from build123d import *

# Parameters (mm, degrees)
SKETCH_1_W          = 32.4
SKETCH_1_H          = 30
EXTRUDE_1_DEPTH     = 1.5
SKETCH_2_W          = 4.9
SKETCH_2_H          = 8.52
EXTRUDE_2_DEPTH     = 10
CUT_EXTRUDE_1_DEPTH = 11.5
SKETCH_4_R          = 1
CUT_EXTRUDE_2_DEPTH = 31.5
CUT_EXTRUDE_3_DEPTH = 10
EXTRUDE_3_DEPTH     = 2
CUT_EXTRUDE_4_DEPTH = 6
SKETCH_8_R          = 2.25
CUT_EXTRUDE_5_DEPTH = 2


with BuildPart() as part:
    # 草图1 → 凸台-拉伸1 (new body)
    with BuildSketch(Plane.XY):
        with Locations((-0.362675268, 2.133428793)):
            Rectangle(SKETCH_1_W, SKETCH_1_H)
    extrude(amount=EXTRUDE_1_DEPTH)

    # 草图2 → 凸台-拉伸2 (add)
    with BuildSketch(Plane.XY.offset(1.5)):
        with Locations((-14.112675268, -1.225199495)):
            Rectangle(SKETCH_2_W, SKETCH_2_H)
        Polygon((-16.562675268, 5.494800505), (-11.662675268, 5.494800505), (-11.662675268, 12.70812694), (-16.562675268, 7.80812694), align=None)
        Polygon((10.937324732, 5.494800505), (10.937324732, 12.70812694), (15.837324732, 7.80812694), (15.837324732, 5.494800505), align=None)
        Polygon((10.937324732, 3.034800505), (15.837324732, 3.034800505), (15.837324732, 0), (10.937324732, -1.245199495), align=None)
    extrude(amount=EXTRUDE_2_DEPTH)

    # 草图3 → 切除-拉伸1 (cut)
    with BuildSketch(Plane.XY.offset(1.5)):
        Polygon((-16.562675268, 7.80812694), (-11.662675268, 12.70812694), (-11.662675268, 17.133428793), (-16.562675268, 17.133428793), align=None)
        Polygon((15.837324732, 7.80812694), (10.937324732, 12.70812694), (10.937324732, 17.133428793), (15.837324732, 17.133428793), align=None)
        Polygon((-16.562675268, -12.866571207), (-16.562675268, -8.702000753), (-16.562675268, -5.485199495), (3.157324732, -5.485199495), (3.157324732, -1.245199495), (10.937324732, -1.245199495), (15.837324732, 0), (15.837324732, -12.866571207), align=None)
    extrude(amount=-CUT_EXTRUDE_1_DEPTH, mode=Mode.SUBTRACT)

    # 草图4 → 切除-拉伸2 (cut)
    with BuildSketch(Plane.XZ.offset(5.485199495)):
        with Locations(Location((-14.162675268, 7.75, 0), (0, 0, 180))):
            Circle(SKETCH_4_R)
        with Locations(Location((13.437324732, 7.75, 0), (0, 0, 270))):
            Circle(SKETCH_4_R)
    extrude(amount=-CUT_EXTRUDE_2_DEPTH, mode=Mode.SUBTRACT)

    # 草图5 → 切除-拉伸3 (cut)
    with BuildSketch(Plane.XY.offset(11.5)):
        with BuildLine():
            Line((-11.662675268, -5.485199495), (-11.662675268, -1.225199495))
            ThreePointArc((-11.662675268, -1.225199495), (-14.426273503, -0.547412969), (-16.562675268, 1.332123483))
            Line((-16.562675268, 1.332123483), (-16.562675268, -5.485199495))
            Line((-16.562675268, -5.485199495), (-11.662675268, -5.485199495))
        make_face()
    extrude(amount=-CUT_EXTRUDE_3_DEPTH, mode=Mode.SUBTRACT)

    # 草图6 → 凸台-拉伸3 (add)
    with BuildSketch(Plane(origin=(0, 0, 0), x_dir=(-1, 0, 0), z_dir=(0, 0, -1))):
        with BuildLine():
            Line((4.562675268, 9.133428793), (7.412675268, 9.133428793))
            ThreePointArc((7.412675268, 9.133428793), (9.412675268, 7.133428793), (7.412675268, 5.133428793))
            Line((7.412675268, 5.133428793), (4.562675268, 5.133428793))
            Line((4.562675268, 5.133428793), (4.562675268, 2.436720349))
            Line((4.562675268, 2.436720349), (11.662675268, 2.436720349))
            Line((11.662675268, 2.436720349), (11.662675268, 11.725210418))
            Line((11.662675268, 11.725210418), (4.562675268, 11.725210418))
            Line((4.562675268, 11.725210418), (4.562675268, 9.133428793))
        make_face()
        with BuildLine():
            Line((-5.287324731, 9.133428793), (-2.437324732, 9.133428793))
            Line((-2.437324732, 9.133428793), (-2.437324732, 11.725210418))
            Line((-2.437324732, 11.725210418), (-10.937324732, 11.725210418))
            Line((-10.937324732, 11.725210418), (-10.937324732, 2.436720349))
            Line((-10.937324732, 2.436720349), (-2.437324732, 2.436720349))
            Line((-2.437324732, 2.436720349), (-2.437324732, 5.133428793))
            Line((-2.437324732, 5.133428793), (-5.287324731, 5.133428793))
            ThreePointArc((-5.287324731, 5.133428793), (-7.287324731, 7.133428793), (-5.287324731, 9.133428793))
        make_face()
    extrude(amount=EXTRUDE_3_DEPTH)

    # 草图7 → 切除-拉伸4 (cut)
    with BuildSketch(Plane.XY.offset(1.5)):
        with BuildLine():
            Line((-16.562675268, 1.332123483), (-16.562675268, -5.485199495))
            Line((-16.562675268, -5.485199495), (-11.683364196, -5.485199495))
            Line((-11.683364196, -5.485199495), (-11.662675268, -1.225199495))
            ThreePointArc((-11.662675268, -1.225199495), (-14.426273503, -0.547412969), (-16.562675268, 1.332123483))
        make_face()
    extrude(amount=-CUT_EXTRUDE_4_DEPTH, mode=Mode.SUBTRACT)

    # 草图8 → 切除-拉伸5 (cut)
    with BuildSketch(Plane.XZ.offset(1.245199495)):
        with Locations((13.437324732, 7.75)):
            Circle(SKETCH_8_R)
        with Locations((-14.162675268, 7.75)):
            Circle(SKETCH_8_R)
    extrude(amount=-CUT_EXTRUDE_5_DEPTH, mode=Mode.SUBTRACT)


solid = part.part
Read the model definition and answer for the solid it produces. Units are mm, in the model's axes. A direction names the side the tool comes from. Coordinates: 2 decimals unless noted, no trailing zeros. Write each loop counter-clockwise with the first axis right and the second up, starting at its lowest first coordinate (ties: lowest second). Pieces come first, ordered by that corner, then holes. Notation, with made-up numbers: (30.5, 50.25) -> (40.5, 50.25) arc R13 ccw to (40.5, 62.25) -> close; hole circle Ø6 at (45.25, -4). An arc over 180 degrees is marked (long way). Return JSON: item names as keys, results as strings.
(1) The part is cut by section C-C on x = 1. Give the vertices of the cut face in (y, z).
Answers below:
{"outline": "(-5.49, 0) -> (17.13, 0) -> (17.13, 1.5) -> (-5.49, 1.5) -> close"}
(2) The part is cut by section A-A on x = 13. Give the vertices of the cut face in (y, z).
Answers below:
{"outline": "(-0.72, 0) -> (10.65, 0) -> (10.65, 6.85) -> (5.49, 6.85) -> (5.49, 1.5) -> (3.03, 1.5) -> (3.03, 6.85) -> (0.75, 6.85) -> (0.75, 5.54) -> (-0.72, 5.54) -> close; (-0.72, 9.96) -> (0.75, 9.96) -> (0.75, 8.65) -> (3.03, 8.65) -> (3.03, 11.5) -> (-0.72, 11.5) -> close; (5.49, 8.65) -> (10.65, 8.65) -> (10.65, 11.5) -> (5.49, 11.5) -> close"}
(3) For a pull along X with two mould halves and no side action, classify faces 4 (the flat face through (10.937, 15, 1)), 5 (the cylindrical face through (-11.914, -0.027, 7.668)), 6 (the cylindrical face through (11.19, -0.03, 7.85)), 7 (the flat face through (-14.15, 10.22, 5.83)) as pulls with the +X half, pulls with the -X half, needs draft (parallel to the pull), parting line crosses it, or undercut.
Answers below:
{"face 4": "pulls with the +X half", "face 5": "undercut", "face 6": "undercut", "face 7": "pulls with the -X half"}
(4) Each of these flat-tipped pins is pushed along its axis until it touches: P1, Ø5.5, axis at x = 14.5, z = 6.5, coming from the +Y side; P2, Ø0.6, axis at y = 4, z = -1.5, coming from the +X side; P3, Ø1, axis at x = -7, z = -1, coming from the +Y side. Where does it stop, or does it pass through?
Answers below:
{"P1": "y = 11.9", "P2": "x = 10.94", "P3": "y = 11.73"}
(5) Consider line 1 along X through (y, z) = (6.5, 3.5); line 2 along Z through (x, y) = (13.5, 3); line 3 along X through (y, z) = (0.1, 7.75). Determine where each line is inside the solid, lowest interval first. Write a range as from..to.
Answers below:
{"line 1": "-16.56..-11.66, 10.94..15.84", "line 2": "0..6.75, 8.75..11.5", "line 3": "-11.91..-11.66, 10.94..11.19, 15.69..15.84"}
(6) Which of the six approach directions +Z, -Z, +X, -X, +Y, -Y give full straight-line access (tool end or side, diameter ignored) to faces 1 (the flat face through (13, 5.495, 6)), 2 (the flat face through (10.937, 7, -1)), 3 (the flat face through (13, 0.755, 9))?
Answers below:
{"face 1": "+Z, +X, -X", "face 2": "-Z, +X, +Y, -Y", "face 3": "-Y"}
(7) The part is cut by section D-D on z = 7.75. State how many separate pieces and enclosed holes the cut face has, then the cut area to 3 significant figures.
Answers below:
{"separate pieces": "8", "enclosed holes": "0", "area": "42.0 mm^2"}
(8) The part is cut by section B-B on y = 4.25. Give the vertices of the cut face in (x, z), then the cut area to 3 significant figures.
Answers below:
{"outline": "(-16.56, 0) -> (-11.66, 0) -> (-11.66, -2) -> (-4.56, -2) -> (-4.56, 0) -> (2.44, 0) -> (2.44, -2) -> (10.94, -2) -> (10.94, 0) -> (15.84, 0) -> (15.84, 1.5) -> (-16.56, 1.5) -> close", "area": "79.8 mm^2"}
